```python
from build123d import *

# Parameters (mm, degrees)
SKETCH1_R           = 3.5
BOSS_EXTRUDE1_DEPTH = 3
SKETCH2_R           = 3.5
BOSS_EXTRUDE2_DEPTH = 3
SKETCH3_W           = 31
SKETCH3_H           = 3
BOSS_EXTRUDE3_DEPTH = 3


with BuildPart() as part:
    # Sketch1 → Boss-Extrude1 (new body)
    with BuildSketch(Plane.XY):
        Circle(SKETCH1_R)
    extrude(amount=BOSS_EXTRUDE1_DEPTH)



with BuildPart() as body_2:
    # Sketch2 → Boss-Extrude2 (new body)
    with BuildSketch(Plane.XY):
        with Locations((31, 0)):
            Circle(SKETCH2_R)
    extrude(amount=BOSS_EXTRUDE2_DEPTH)


with BuildPart() as part_1:
    add(part.part)

    add(body_2.part)  # Boss-Extrude3 merges body 2
    # Sketch3 → Boss-Extrude3 (add)
    with BuildSketch(Plane.XY):
        with Locations((15.5, 0)):
            Rectangle(SKETCH3_W, SKETCH3_H)
    extrude(amount=BOSS_EXTRUDE3_DEPTH)


solid = part_1.part
```
Input: part model. Units: mm. Frame: model coordinates. A direction names the side the tool comes from. Round coordinates to 2 decimals unless told otherwise and drop trailing zeros. Order: outer loops, then holes, each group sorted by start corner. A loop starts at its lowest first (then second) coordinate and runs counter-clockwise, first axis right, second up. Notation, with made-up numbers: (64.25, 61.25) - (98.25, 61.25) arc R21 ccw to (98.25, 85.25) - close; hole circle Ø4 at (-12, 81.25). An arc over 180 degrees is marked (long way). One line per question, with ' | ' between items. Start each with the question number.
1) Set-up query: faces 1 (the flat face through (15, 1.5, 1)), 2 (the flat face through (15, -1.5, 1)), 3 (the cylindrical face through (34.5, -0.1, 1.5)). Return all of +Z, -Z, +X, -X, +Y, -Y with unobstructed straight access to the full face (end or side cutting, diameter ignored); none if empty.
2) Cut plane B-B, the plane z = 1.6. Return the cut outline in (x, y), then the cut area to 3 significant figures.
3) Cut plane D-D, the plane y = 2.5. Return the cut outline in (x, z).
4) Cut plane A-A, the plane y = -2. Return the cut outline in (x, z).
5) Ray query, probe 1 along Y at (x, z) = (12, 0.1); probe 2 along X at (y, z) = (-2, 0.65); probe 3 along X at (y, z) = (-3, 1.2). Return the intervals inside material, ascending.
6) Cut plane C-C, the plane x = 20. Return the cut outline in (y, z), then the cut area to 3 significant figures.
Worked out:
1) face 1: +Z, -Z, +Y | face 2: +Z, -Z, -Y | face 3: +Z, -Z
2) outline: (3.16, -1.5) - (27.84, -1.5) arc R3.5 ccw (long way) to (27.84, 1.5) - (3.16, 1.5) arc R3.5 ccw (long way) to start | area: 150 mm^2
3) outline: (-2.45, 0) - (2.45, 0) - (2.45, 3) - (-2.45, 3) - close; (28.55, 0) - (33.45, 0) - (33.45, 3) - (28.55, 3) - close
4) outline: (-2.87, 0) - (2.87, 0) - (2.87, 3) - (-2.87, 3) - close; (28.13, 0) - (33.87, 0) - (33.87, 3) - (28.13, 3) - close
5) probe 1: y = -1.5 to 1.5 | probe 2: x = -2.87 to 2.87, 28.13 to 33.87 | probe 3: x = -1.8 to 1.8, 29.2 to 32.8
6) outline: (-1.5, 0) - (1.5, 0) - (1.5, 3) - (-1.5, 3) - close | area: 9.00 mm^2
